The listing builds one solid part. Answer for the finished solid, in the listing's coordinates (mm). A direction names the side the tool comes from. Coordinates: 2 decimals unless noted, no trailing zeros. Write each loop counter-clockwise with the first axis right and the second up, starting at its lowest first coordinate (ties: lowest second). Pieces come first, ordered by that corner, then holes.
from build123d import *

# Parameters (mm, degrees)
F0_R     = 16.891
F0_R_2   = 3.3655
F1_DEPTH = 17.272
F2_R     = 1.5875
F2_R_2   = 2.667
F3_DEPTH = 25.4
F5_DEPTH = 5.08


with BuildPart() as f1:
    # F0 (on Top) → F1 (new body)
    with BuildSketch(Plane.XY):
        Circle(F0_R)
        Circle(F0_R_2, mode=Mode.SUBTRACT)
    extrude(amount=F1_DEPTH)

    # F2 (on face) → F3 (cut)
    with BuildSketch(Plane.XY.offset(17.272)):
        with Locations((14.0208, 0)):
            Circle(F2_R)
        with Locations((-12.7508, 0)):
            Circle(F2_R_2)
    extrude(amount=-F3_DEPTH, mode=Mode.SUBTRACT)

    # F4 (on face) → F5 (cut)
    with BuildSketch(Plane(origin=(0, 0, 0), x_dir=(1, 0, 0), z_dir=(0, 0, -1))):
        with BuildLine():
            ThreePointArc((0, -9.652), (-9.652, 0), (0, 9.652))
            ThreePointArc((0, 9.652), (3.740685, 12.7762), (0, 15.9004))
            ThreePointArc((0, 15.9004), (-15.9004, 0), (0, -15.9004))
            ThreePointArc((0, -15.9004), (2.609315, -12.7762), (0, -9.652))
        make_face()
    extrude(amount=-F5_DEPTH, mode=Mode.SUBTRACT)


solid = f1.part
Q1. The part is cut by section D-D, the plane y = 6. Write down the section's boundary in (x, z).
Answers below:
outline: (-15.79, 0) - (-14.72, 0) - (-14.72, 5.08) - (-7.56, 5.08) - (-7.56, 0) - (15.79, 0) - (15.79, 17.27) - (-15.79, 17.27) - close
Q2. Which of the six approach directions +Z, -Z, +X, -X, +Y, -Y give full straight-line access (tool end or side, diameter ignored) to faces 4 (the face through (-15.897, -0.35, 2.504)), 5 (the face through (4, 0, 0))?
Answers below:
face 4: -Z
face 5: -Z, +X, -X, +Y, -Y
Q3. Find the intervals of material crossed by probe 1 along Y at (x, z) = (1, 2); probe 2 along Y at (x, z) = (0, 10.5); probe 3 along Z at (x, y) = (-11.5, 9.5), in increasing order.
Answers below:
probe 1: y = -16.86 to -15.92, -9.63 to -3.21, 3.21 to 10.01, 15.54 to 16.86
probe 2: y = -16.89 to -3.37, 3.37 to 16.89
probe 3: z = 5.08 to 17.27
Q4. Determine the mould class of faces 1 (the face through (16.111, 5.074, 8.515)), 2 (the face through (-11, -4, 5.08)), 3 (the face through (4, 0, 17.272)) for opening direction Y: released by +Y, released by -Y, zero draft, split by the parting line, or undercut.
Answers below:
face 1: split by the parting line
face 2: undercut
face 3: zero draft
Q5. The part is cut by section B-B, the plane z = 4.5. State how many separate pieces and enclosed holes the cut face has, then the cut area to 3 significant figures.
Answers below:
separate pieces: 1
enclosed holes: 3
area: 570 mm2
Q6. The part is cut by section C-C, the plane x = -2. Write down the section's boundary in (y, z).
Answers below:
outline: (-16.77, 0) - (-15.77, 0) - (-15.77, 5.08) - (-9.44, 5.08) - (-9.44, 0) - (-2.71, 0) - (-2.71, 17.27) - (-16.77, 17.27) - close; (2.71, 0) - (9.44, 0) - (9.44, 5.08) - (15.77, 5.08) - (15.77, 0) - (16.77, 0) - (16.77, 17.27) - (2.71, 17.27) - close
Q7. The part is cut by section A-A, the plane y = 0. Write down the section's boundary in (x, z).
Answers below:
outline: (-16.89, 0) - (-15.9, 0) - (-15.9, 5.08) - (-15.42, 5.08) - (-15.42, 17.27) - (-16.89, 17.27) - close; (-10.08, 5.08) - (-9.65, 5.08) - (-9.65, 0) - (-3.37, 0) - (-3.37, 17.27) - (-10.08, 17.27) - close; (3.37, 0) - (12.43, 0) - (12.43, 17.27) - (3.37, 17.27) - close; (15.61, 0) - (16.89, 0) - (16.89, 17.27) - (15.61, 17.27) - close
Q8. Given pin 1 (3 mm diameter, centred on x = -7.5, z = 8.5, fed in from +Y); pin 2 (5 mm diameter, centred on x = -12.75, y = 0, fed in from -Z); pin 3 (1 mm diameter, centred on y = -11, z = 15, fed in from -X); pin 4 (3 mm diameter, centred on x = 5.5, z = 13, fed in from +Y), each flat-ended and moving along its own axis, determine where each tip first touches the part or whether it passes through.
Answers below:
pin 1: stops at y = 15.79
pin 2: passes through
pin 3: stops at x = -13.23
pin 4: stops at y = 16.41
